Part model, mm, in its own coordinate system. Round coordinates to 2 decimals unless told otherwise and drop trailing zeros. Write each loop counter-clockwise with the first axis right and the second up, starting at its lowest first coordinate (ties: lowest second). Pieces come first, ordered by that corner, then holes. Notation, with made-up numbers: M 77,84 L 135,84 A12 cw 135,95 Z; hole C 70.25,-5.5 d11. An arc over 180 degrees is marked long. Use one line per item in the form item = value. Start each with the question number.
Item 1: Cut at A-A, the plane y = 0. Give the cut face in (x, z), then the cut area to 3 significant figures.
Item 2: Flat gauge pins, fed straight in: pin 1 Ø1 at (x, y) = (2, 4) entering from +Z; pin 2 Ø1 at (x, z) = (3.5, 11.5) entering from -Y. Where does each tip first touch, or does it go through?
Item 3: Probe L1, parallel to Y at x = 1.8, z = 0; L2, parallel to Z at x = 1.4, y = 0.5; L3, parallel to Z at x = 1.95, y = -12.5. List the from-to ranges inside material, lowest first.
from build123d import *

# Parameters (mm, degrees)
ESQUISSE1_W = 4
ESQUISSE1_H = 5
CONG_1_R    = 1


with BuildPart() as part:
    # Esquisse1 → Base-Révolution (revolve)
    with BuildSketch(Plane.XY, mode=Mode.PRIVATE) as base_r_volution_sk:
        with Locations((2, 17.5)):
            Rectangle(ESQUISSE1_W, ESQUISSE1_H)
    revolve(base_r_volution_sk.sketch.rotate(Axis((0, 0, 0), (-1, 0, 0)), 90), axis=Axis((0, 0, 0), (-1, 0, 0)))

    # Congé1
    cong_1_edges = [part.edges().sort_by_distance(p)[0] for p in [
        (0, 0, 15),
        (4, 0, 15),
        (4, 0, 20),
        (0, 0, 20),
    ]]
    fillet(cong_1_edges, radius=CONG_1_R)


solid = part.part
Model answer:
q1.outline = M 0,-19 A1 ccw 1,-20 L 3,-20 A1 ccw 4,-19 L 4,-16 A1 ccw 3,-15 L 1,-15 A1 ccw 0,-16 Z; M 0,16 A1 ccw 1,15 L 3,15 A1 ccw 4,16 L 4,19 A1 ccw 3,20 L 1,20 A1 ccw 0,19 Z
q1.area = 38.3 mm²
q2.pin_1 = 19.69
q2.pin_2 = -16.62
q3.L1 = -20 to -15, 15 to 20
q3.L2 = -19.99 to -14.99, 14.99 to 19.99
q3.L3 = -15.61 to -8.29, 8.29 to 15.61
